For this review, take the finished solid that the model builds, in its own axes (mm). A direction names the side the tool comes from. Round coordinates to 2 decimals unless told otherwise and drop trailing zeros. Write each loop counter-clockwise with the first axis right and the second up, starting at its lowest first coordinate (ties: lowest second). Pieces come first, ordered by that corner, then holes. Notation, with made-up numbers: (-38.5, 47) - (-30.5, 47) arc R6 cw to (-30.5, 54) - close; hole circle Ø4 at (47, -8.75). An arc over 180 degrees is marked (long way). One line per item, written item: value. Start each with the question number.
Q1. Add section A-A on y = 0. Write out the cut boundary in (x, z).
Q2. Add section B-B on z = -0.75. Write out the cut boundary in (x, y), and give its area (3 significant figures).
Q3. Clearance check with flat-ended pins moving along their axes: pin 1 Ø1 at (x, y) = (-10.5, -2) entering from -Z; pin 2 Ø0.8 at (y, z) = (2.5, -0.5) entering from -X; pin 3 Ø1.8 at (x, y) = (17, 0) entering from -Z; pin 4 Ø3 at (x, z) = (-6, 2) entering from +Y. State where each tip first meets the part, or that it passes through.
Q4. Add section D-D on x = 8. Write out the cut boundary in (y, z).
Q5. For probe 1 along X at (y, z) = (0, 0.9); probe 2 along X at (y, z) = (-1, 1); probe 3 along Y at (x, z) = (17, -1.2), list the stretches that pass through material, from the lowest coordinate up.
Q6. Add section C-C on x = 17. Write out the cut boundary in (y, z), and give its area (3 significant figures).
Q7. Tool access review of faces 1 (the face through (16, 2.25, 0)), 2 (the face through (-17, -2.25, 0)), 3 (the face through (-17, 2.25, 0)): name each direction out of +Z, -Z, +X, -X, +Y, -Y from which nothing blocks a thin tool from reaching the whole face with its end or side.
```python
from build123d import *

# Parameters (mm, degrees)
SKETCH1_W               = 40
SKETCH1_H               = 3
SKETCH2_W               = 7
SKETCH2_H               = 0.75
CUT_EXTRUDE1_DEPTH      = 4
CUT_EXTRUDE1_DEPTH_BACK = 4
SKETCH3_R               = 1.1
CUT_EXTRUDE2_DEPTH      = 4
CUT_EXTRUDE2_DEPTH_BACK = 4


with BuildPart() as part:
    # Sketch1 → Revolve1 (revolve)
    with BuildSketch(Plane.XY):
        with Locations((0, 1.5)):
            Rectangle(SKETCH1_W, SKETCH1_H)
    revolve(axis=Axis((0, 0, 0), (1, 0, 0)))

    # Sketch2 → Cut-Extrude1 (cut, two sides)
    with BuildSketch(Plane.XY) as cut_extrude1_sk:
        with Locations((-16.5, 2.625)):
            Rectangle(SKETCH2_W, SKETCH2_H)
        with Locations((-16.5, -2.625)):
            Rectangle(SKETCH2_W, SKETCH2_H)
        with Locations((16.5, 2.625)):
            Rectangle(SKETCH2_W, SKETCH2_H)
        with Locations((16.5, -2.625)):
            Rectangle(SKETCH2_W, SKETCH2_H)
    extrude(amount=CUT_EXTRUDE1_DEPTH, mode=Mode.SUBTRACT)
    extrude(cut_extrude1_sk.sketch, amount=-CUT_EXTRUDE1_DEPTH_BACK, mode=Mode.SUBTRACT)

    # Sketch3 → Cut-Extrude2 (cut, two sides)
    with BuildSketch(Plane.XY) as cut_extrude2_sk:
        with Locations((-17, 0)):
            Circle(SKETCH3_R)
        with Locations((17, 0)):
            Circle(SKETCH3_R)
    extrude(amount=CUT_EXTRUDE2_DEPTH, mode=Mode.SUBTRACT)
    extrude(cut_extrude2_sk.sketch, amount=-CUT_EXTRUDE2_DEPTH_BACK, mode=Mode.SUBTRACT)


solid = part.part
```
Result set:
1. outline: (-20, -3) - (-18.1, -3) - (-18.1, 3) - (-20, 3) - close; (-15.9, -3) - (15.9, -3) - (15.9, 3) - (-15.9, 3) - close; (18.1, -3) - (20, -3) - (20, 3) - (18.1, 3) - close
2. outline: (-20, -2.25) - (-13, -2.25) - (-13, -2.9) - (13, -2.9) - (13, -2.25) - (20, -2.25) - (20, 2.25) - (13, 2.25) - (13, 2.9) - (-13, 2.9) - (-13, 2.25) - (-20, 2.25) - close; hole circle Ø2.2 at (-17, 0); hole circle Ø2.2 at (17, 0)
2. area: 206 mm^2
3. pin 1: stops at z = -2.6
3. pin 2: stops at x = -20
3. pin 3: passes through
3. pin 4: stops at y = 2.96
4. outline: circle Ø6 at (0, 0)
5. probe 1: x = -20 to -18.1, -15.9 to 15.9, 18.1 to 20
5. probe 2: x = -20 to -17.46, -16.54 to 16.54, 17.46 to 20
5. probe 3: y = -2.25 to -1.1, 1.1 to 2.25
6. outline: (-2.25, -1.98) arc R3 ccw to (-1.1, -2.79) - (-1.1, 2.79) arc R3 ccw to (-2.25, 1.98) - close; (1.1, -2.79) arc R3 ccw to (2.25, -1.98) - (2.25, 1.98) arc R3 ccw to (1.1, 2.79) - close
6. area: 11.3 mm^2
7. face 1: +Z, -Z, +X, +Y
7. face 2: +Z, -Z, -X, -Y
7. face 3: +Z, -Z, -X, +Y
